Input: dimensioned drawing with shaded views. Units: mm. Origin: part minimum x, y, z. Give positions to 0.01 mm unless a question says otherwise; leave off trailing zeros. Order: outer loops, then holes, each group sorted by start corner. A loop starts at its lowest first (then second) coordinate and runs counter-clockwise, first axis right, second up.
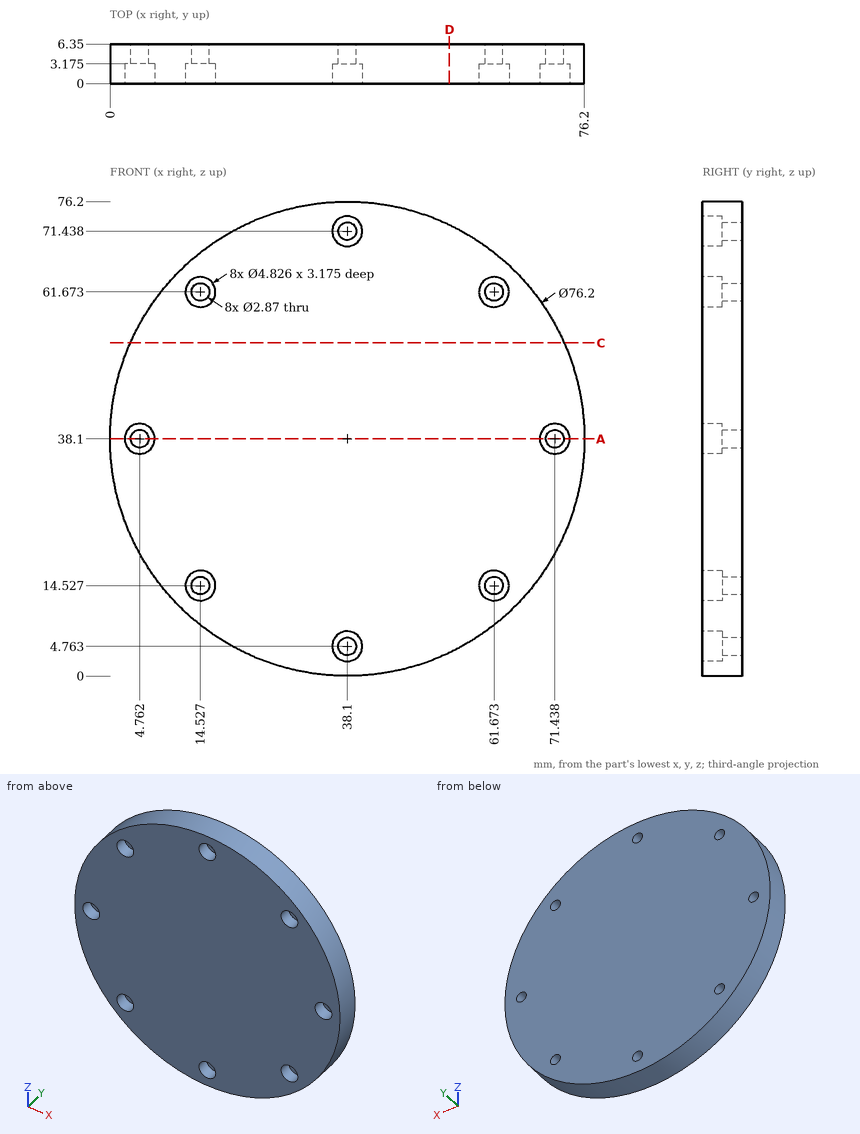
1) Pin query (flat end, axial travel): pin 1 (3 mm diameter, centred on x = 56.5, z = 13.5, fed in from -Y); pin 2 (2.5 mm diameter, centred on x = 15, z = 14, fed in from -Y) (1 decimal); pin 3 (1.7 mm diameter, centred on x = 14.53, z = 61.67, fed in from +Y); pin 4 (2 mm diameter, centred on y = 1, z = 58.5, fed in from -X). Return the tip coordinate at first contact, or that it passes through.
Report:
pin 1: stops at y = 0
pin 2: stops at y = 3.2
pin 3: passes through
pin 4: stops at x = 5.31
2) Section query A-A, the plane z = 38.1. Count the separate pieces of the cut face and the enclosed holes in it, and give its area (3 significant figures).
Report:
separate pieces: 3
enclosed holes: 0
area: 435 mm2
3) Section query C-C, the plane z = 53.5. Return the cut outline in (x, y).
Report:
outline: (3.25, 0) - (72.95, 0) - (72.95, 6.35) - (3.25, 6.35) - close
4) Material intervals for L1, parallel to X at y = 4.95, z = 38.1; L2, parallel to X at y = 2, z = 60 (1 decimal); L3, parallel to Z at x = 14, y = 6, sorted ascending.
Report:
L1: x = 0 to 3.33, 6.2 to 70, 72.87 to 76.2
L2: x = 6.9 to 12.8, 16.3 to 59.9, 63.4 to 69.3
L3: z = 8.59 to 13.19, 15.86 to 60.34, 63.01 to 67.61
5) Section query D-D, the plane x = 54.5. Return the cut outline in (y, z).
Report:
outline: (0, 3.71) - (6.35, 3.71) - (6.35, 72.49) - (0, 72.49) - close
